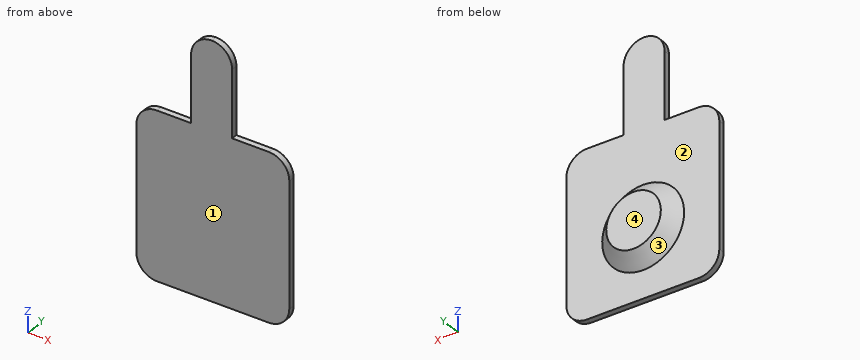
```python
from build123d import *

# Parameters (mm, degrees)
SKETCH1_W           = 11.2
SKETCH1_H           = 12
SKETCH1_W_2         = 3
SKETCH1_H_2         = 6.34
BOSS_EXTRUDE1_DEPTH = 0.45
FILLET1_R           = 1.5
SKETCH2_R           = 2
BOSS_EXTRUDE2_DEPTH = 1
CHAMFER1_SIZE       = 1


with BuildPart() as part:
    # Sketch1 → Boss-Extrude1 (new body)
    with BuildSketch(Plane(origin=(0, 0, 0), x_dir=(1, 0, 0), z_dir=(0, 1, 0))):
        with Locations((5.6, 6)):
            Rectangle(SKETCH1_W, SKETCH1_H)
        with Locations((5.509745164, -3.17)):
            Rectangle(SKETCH1_W_2, SKETCH1_H_2)
    extrude(amount=BOSS_EXTRUDE1_DEPTH)

    # Fillet1
    fillet1_edges = [part.edges().sort_by_distance(p)[0] for p in [
        (0, 0.225, 0),
        (0, 0.225, -12),
        (11.2, 0.225, -12),
        (11.2, 0.225, 0),
        (7.009745164, 0.225, 6.34),
        (4.009745164, 0.225, 6.34),
    ]]
    fillet(fillet1_edges, radius=FILLET1_R - 0.0001)  # a hair under: the kernel refuses the full size

    # Sketch2 → Boss-Extrude2 (add)
    with BuildSketch(Plane(origin=(0, 0.45, 0), x_dir=(1, 0, 0), z_dir=(0, 1, 0))):
        with Locations(Location((5.575393992, 7, 0), (0, 0, 270))):
            Circle(SKETCH2_R)
    extrude(amount=BOSS_EXTRUDE2_DEPTH)

    # Chamfer1
    chamfer1_edges = [part.edges().sort_by_distance(p)[0] for p in [
        (5.575393992, 0.45, -9),
    ]]
    chamfer(chamfer1_edges, length=CHAMFER1_SIZE - 0.0001)  # a hair under: the kernel refuses the full size


solid = part.part
```
Verification items for the finished model (mm, model axes). Face numbers are marked on the shaded views. A direction names the side the tool comes from. Coordinates: 2 decimals unless noted, no trailing zeros. Loops run counter-clockwise (first coordinate to the right, second up) from the corner with the lowest first, then second, coordinate; pieces in that order, holes last. Notation, with made-up numbers: (-29, 74.5) -> (3, 74.5) arc R25 ccw to (3, 103.5) -> close; hole circle Ø5 at (88.5, 24). An arc over 180 degrees is marked (long way). Answer in a Markdown table with one row per item.
1) Scan lines: line 1 along X through (y, z) = (0.2, 4.5); line 2 along Y through (x, z) = (10.5, -5.5); line 3 along X through (y, z) = (0.65, -6). Record each from-to range of solid material in increasing order. Write a range as from..to.
The answers:
| item | result |
|---|---|
| line 1 | x = 4.01..7.01 |
| line 2 | y = 0..0.45 |
| line 3 | x = 2.96..8.19 |
2) Draft check along X on the marked faces 3 and 4. Enter one of: released by +X, released by -X, zero draft, split by the parting line, or undercut.
The answers:
| item | result |
|---|---|
| face 3 | split by the parting line |
| face 4 | zero draft |
3) Section check C-C (z = 4). Record the cut outline in (x, y).
The answers:
| item | result |
|---|---|
| outline | (4.01, 0) -> (7.01, 0) -> (7.01, 0.45) -> (4.01, 0.45) -> close |
4) Depth check by flat-ended pin: P1, Ø0.5, axis at y = 0.5, z = 1.5, coming from the -X side; P2, Ø0.5, axis at y = 0.5, z = 2.5, coming from the +X side. Enter the tip coordinate at first touch or a pass-through.
The answers:
| item | result |
|---|---|
| P1 | stops at x = 4.01 |
| P2 | stops at x = 7.01 |
5) Access from +Z, -Z, +X, -X, +Y, -Y to the whole of each face (thin tool, end or side, straight path). Record for the marked faces 1 and 2.
The answers:
| item | result |
|---|---|
| face 1 | +Z, -Z, +X, -X, -Y |
| face 2 | +Y |
6) Section check B-B (y = 1.2). Record the cut outline in (x, z), and give its area (3 significant figures).
The answers:
| item | result |
|---|---|
| outline | circle Ø4.5 at (5.58, -7) |
| area | 15.9 mm2 |
